Here's how the part is built. I have some questions about the finished solid (model axes, mm). Give positions to 0.01 mm unless a question says otherwise; leave off trailing zeros. Loops run counter-clockwise (first coordinate to the right, second up) from the corner with the lowest first, then second, coordinate; pieces in that order, holes last.
Q1. Suppose I cut it at B-B (y = -126.5). List the corners of the cut face in (x, z) for me, and give its area (3 significant figures).
Q2. Suppose I cut it at A-A (y = -40). List the corners of the cut face in (x, z) for me, and give its area (3 significant figures).
Q3. I need wall thicknesses on probe 1 along X at (y, z) = (3, 0.5); probe 2 along X at (y, z) = (-42.5, 4.25); probe 3 along Z at (x, y) = (6.25, -66.5). Which ranges of each line are inside material? Lowest first, please.
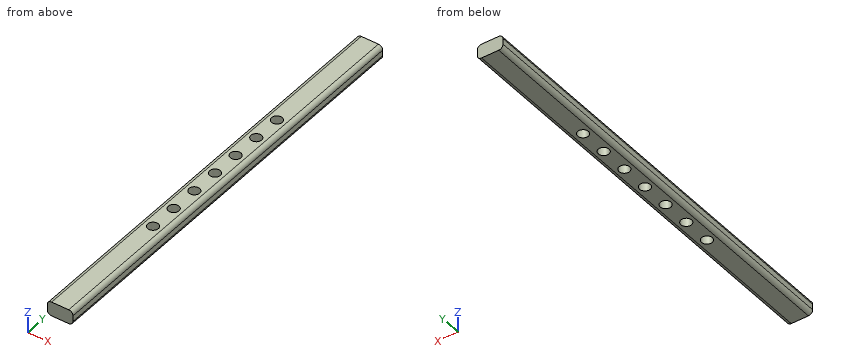
```python
from build123d import *

# Parameters (mm, degrees)
CROQUIS1_W              = 18
CROQUIS1_H              = 300
SALIENTE_EXTRUIR1_DEPTH = 5
REDONDEO2_R             = 3
CROQUIS2_R              = 3.747917417
CORTAR_EXTRUIR1_DEPTH   = 10


with BuildPart() as part:
    # Croquis1 → Saliente-Extruir1 (new, symmetric)
    with BuildSketch(Plane.XY):
        Rectangle(CROQUIS1_W, CROQUIS1_H)
    extrude(amount=SALIENTE_EXTRUIR1_DEPTH, both=True)

    # Redondeo2
    redondeo2_edges = [part.edges().sort_by_distance(p)[0] for p in [
        (-9, 0, 5),
        (9, 0, 5),
        (-9, 0, -5),
        (9, 0, -5),
    ]]
    fillet(redondeo2_edges, radius=REDONDEO2_R)

    # Croquis2 → Cortar-Extruir1 (cut)
    with BuildSketch(Plane.XY.offset(5)):
        Circle(CROQUIS2_R)
        with Locations((0, 20)):
            Circle(CROQUIS2_R)
        with Locations((0, 40)):
            Circle(CROQUIS2_R)
        with Locations((0, 60)):
            Circle(CROQUIS2_R)
        with Locations((0, -20)):
            Circle(CROQUIS2_R)
        with Locations((0, -60)):
            Circle(CROQUIS2_R)
        with Locations((0, -40)):
            Circle(CROQUIS2_R)
    extrude(amount=-CORTAR_EXTRUIR1_DEPTH, mode=Mode.SUBTRACT)


solid = part.part
```
Solutions:
1. outline: (-9, -2) arc R3 ccw to (-6, -5) - (6, -5) arc R3 ccw to (9, -2) - (9, 2) arc R3 ccw to (6, 5) - (-6, 5) arc R3 ccw to (-9, 2) - close
1. area: 172 mm2
2. outline: (-9, -2) arc R3 ccw to (-6, -5) - (-3.75, -5) - (-3.75, 5) - (-6, 5) arc R3 ccw to (-9, 2) - close; (3.75, -5) - (6, -5) arc R3 ccw to (9, -2) - (9, 2) arc R3 ccw to (6, 5) - (3.75, 5) - close
2. area: 97.3 mm2
3. probe 1: x = -9 to -2.25, 2.25 to 9
3. probe 2: x = -7.98 to -2.79, 2.79 to 7.98
3. probe 3: z = -4.99 to 4.99
